Answer from the drawing. Dimensions are ordinates in mm from the lowest x, y and z of the part. Round coordinates to 2 decimals unless told otherwise and drop trailing zeros. Order: outer loops, then holes, each group sorted by start corner. A loop starts at its lowest first (then second) coordinate and runs counter-clockwise, first axis right, second up.
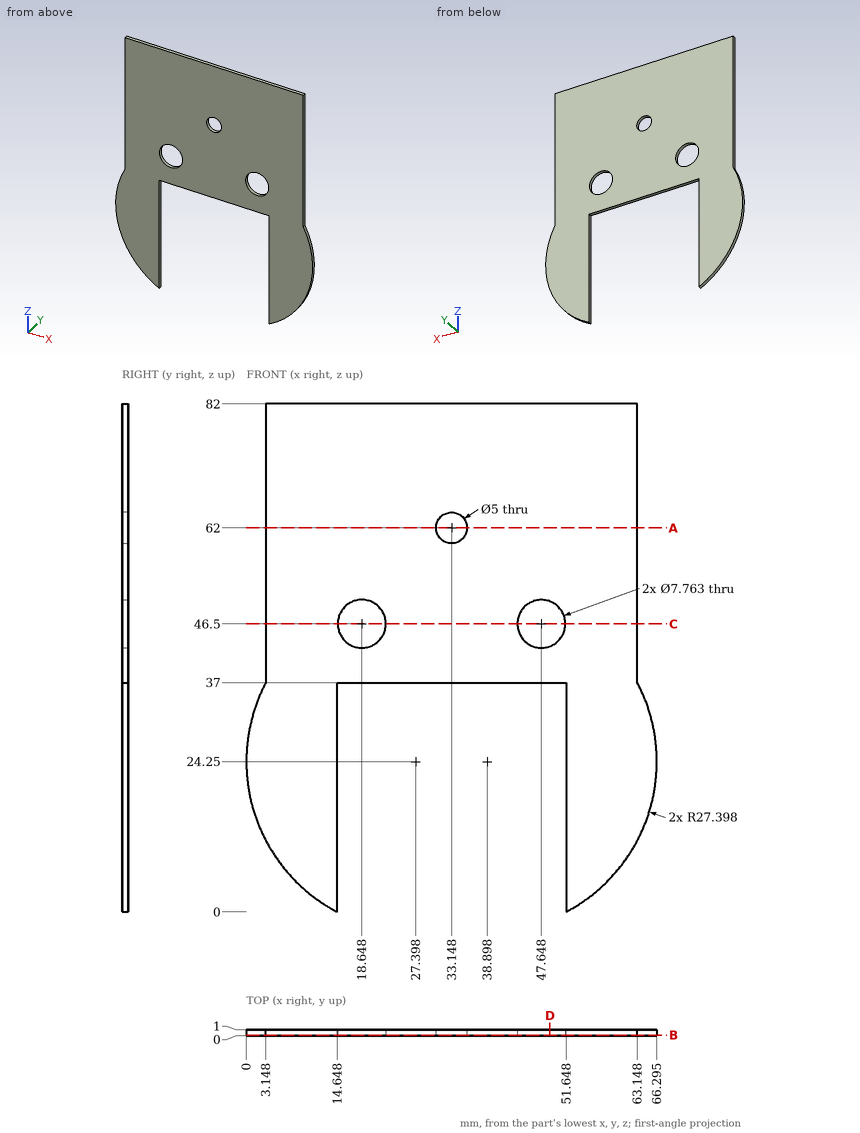
Q1. A cutting plane is placed at C-C, the plane z = 46.5. Give the vertices of the cut face in (x, y).
Outcome:
outline: (3.15, 0) - (14.77, 0) - (14.77, 1) - (3.15, 1) - close; (22.53, 0) - (43.77, 0) - (43.77, 1) - (22.53, 1) - close; (51.53, 0) - (63.15, 0) - (63.15, 1) - (51.53, 1) - close
Q2. Straight lines are drawn through the part: probe 1 along X at (y, z) = (0.5, 46.5); probe 2 along X at (y, z) = (0.4, 65); probe 3 along Z at (x, y) = (50.5, 0.6) (1 decimal). For each, find the intervals that lie inside material, in ascending order.
Outcome:
probe 1: x = 3.15 to 14.77, 22.53 to 43.77, 51.53 to 63.15
probe 2: x = 3.15 to 63.15
probe 3: z = 37 to 43.9, 49.1 to 82
Q3. A cutting plane is placed at B-B, the plane y = 0.15. Give the number of separate pieces and of enclosed holes in the cut face, plus the area to 3 significant figures.
Outcome:
separate pieces: 1
enclosed holes: 3
area: 3,440 mm2
Q4. A flat-ended cylindrical pin translates along its axis: pin 1 (3 mm diameter, centred on x = 33.15, z = 62, fed in from +Y). Find the tip coordinate at first contact, or state that the pin passes through.
Outcome:
pin 1: passes through
Q5. A cutting plane is placed at D-D, the plane x = 49. Give the vertices of the cut face in (y, z).
Outcome:
outline: (0, 37) - (1, 37) - (1, 42.86) - (0, 42.86) - close; (0, 50.14) - (1, 50.14) - (1, 82) - (0, 82) - close
Q6. A cutting plane is placed at A-A, the plane z = 62. Give the vertices of the cut face in (x, y).
Outcome:
outline: (3.15, 0) - (30.65, 0) - (30.65, 1) - (3.15, 1) - close; (35.65, 0) - (63.15, 0) - (63.15, 1) - (35.65, 1) - close
